CAD build for the part. Positions are in the model's coordinates, mm. Face numbers are marked on the shaded views. Coordinates: 2 decimals unless noted, no trailing zeros. Loops run counter-clockwise (first coordinate to the right, second up) from the corner with the lowest first, then second, coordinate; pieces in that order, holes last. Notation, with made-up numbers: (29.5, 14.5) - (60.5, 14.5) arc R21 cw to (60.5, 19.5) - close; hole circle Ø4 at (-25, 8.25). An arc over 180 degrees is marked (long way). Put each result on its own line as item: value.
```python
from build123d import *

# Parameters (mm, degrees)
BOSS_EXTRUDE1_DEPTH = 3.175
CUT_EXTRUDE1_REACH  = 8.35
SKETCH2_R           = 7.14375


with BuildPart() as part:
    # Sketch1 → Boss-Extrude1 (new body, symmetric)
    with BuildSketch(Plane(origin=(0, 0, 0), x_dir=(0, 0, -1), z_dir=(1, 0, 0))):
        with BuildLine():
            Line((-15.875, -28.575), (-15.875, 28.575))
            ThreePointArc((-15.875, 28.575), (0, 44.45), (15.875, 28.575))
            Line((15.875, 28.575), (15.875, -28.575))
            ThreePointArc((15.875, -28.575), (0, -44.45), (-15.875, -28.575))
        make_face()
    extrude(amount=BOSS_EXTRUDE1_DEPTH, both=True)

    # Sketch2 → Cut-Extrude1 (cut, up to next)
    with BuildSketch(Plane(origin=(3.175, 0, 0), x_dir=(0, 0, -1), z_dir=(1, 0, 0)), mode=Mode.PRIVATE) as cut_extrude1_sk1:
        with Locations((0, 28.575)):
            Circle(SKETCH2_R)
    cut_extrude1_tool1 = extrude(cut_extrude1_sk1.sketch, amount=-CUT_EXTRUDE1_REACH, mode=Mode.PRIVATE) & part.part
    add(cut_extrude1_tool1.solids().sort_by_distance((3.175, 28.575, 0))[0], mode=Mode.SUBTRACT)
    # Sketch2 → Cut-Extrude1 (cut, up to next)
    with BuildSketch(Plane(origin=(3.175, 0, 0), x_dir=(0, 0, -1), z_dir=(1, 0, 0)), mode=Mode.PRIVATE) as cut_extrude1_sk2:
        with Locations((0, -28.575)):
            Circle(SKETCH2_R)
    cut_extrude1_tool2 = extrude(cut_extrude1_sk2.sketch, amount=-CUT_EXTRUDE1_REACH, mode=Mode.PRIVATE) & part.part
    add(cut_extrude1_tool2.solids().sort_by_distance((3.175, -28.575, 0))[0], mode=Mode.SUBTRACT)


solid = part.part
```
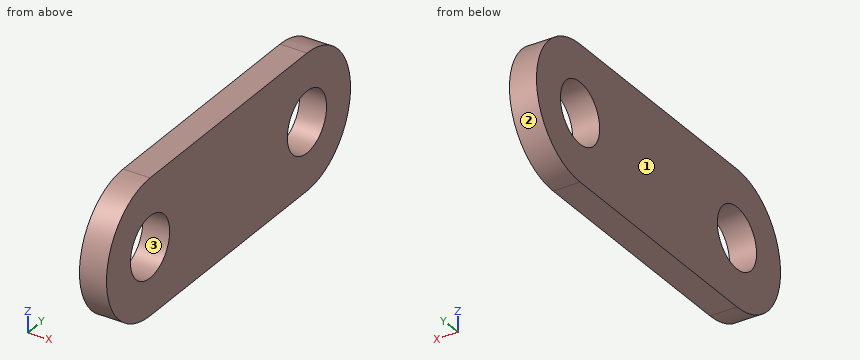
Q1. Pin check, flat tip, straight feed: pin 1 Ø10 at (y, z) = (-30.5, -6.5) entering from +X (3 decimals). Stop position of the tip, or through.
Determined:
pin 1: x = 3.175
Q2. Slice it at A-A, the plane z = 0. Give the cut face in (x, y) (3 decimals), then the cut area to 3 significant figures.
Determined:
outline: (-3.175, -44.45) - (3.175, -44.45) - (3.175, -35.719) - (-3.175, -35.719) - close; (-3.175, -21.431) - (3.175, -21.431) - (3.175, 21.431) - (-3.175, 21.431) - close; (-3.175, 35.719) - (3.175, 35.719) - (3.175, 44.45) - (-3.175, 44.45) - close
area: 383 mm2
Q3. Wall check: L1, parallel to Y at x = 0.75, z = 0; L2, parallel to Y at x = 2.25, z = -5.5; L3, parallel to Z at x = 0, y = -31. Give the ranges that are in metal, low to high. Write a range as from..to.
Determined:
L1: -44.45..-35.72, -21.43..21.43, 35.72..44.45
L2: -43.47..-33.13, -24.02..24.02, 33.13..43.47
L3: -15.69..-6.72, 6.72..15.69
Q4. Slice it at C-C, the plane z = 6. Give the cut face in (x, y) (3 decimals), then the cut area to 3 significant figures.
Determined:
outline: (-3.175, -43.272) - (3.175, -43.272) - (3.175, -32.452) - (-3.175, -32.452) - close; (-3.175, -24.698) - (3.175, -24.698) - (3.175, 24.698) - (-3.175, 24.698) - close; (-3.175, 32.452) - (3.175, 32.452) - (3.175, 43.272) - (-3.175, 43.272) - close
area: 451 mm2
Q5. Slice it at B-B, the plane x = -0.25. State how many separate pieces and enclosed holes the cut face has, then the cut area to 3 significant figures.
Determined:
separate pieces: 1
enclosed holes: 2
area: 2,290 mm2
Q6. Mould opens along Z. For the marked faces 1, 2 and 3 say: +Z half, -Z half, draft (parallel to the pull), parting line (faces both ways), or undercut.
Determined:
face 1: draft
face 2: parting line
face 3: undercut
Q7. Slice it at D-D, the plane z = 10.5. Give the cut face in (x, y) (3 decimals).
Determined:
outline: (-3.175, -40.482) - (3.175, -40.482) - (3.175, 40.482) - (-3.175, 40.482) - close
